Input: part model. Units: mm. Frame: model coordinates. Face numbers are marked on the shaded views. A direction names the side the tool comes from. Round coordinates to 2 decimals unless told otherwise and drop trailing zeros. Loops run counter-clockwise (first coordinate to the right, second up) from the corner with the lowest first, then second, coordinate; pieces in that order, holes last. Notation, with made-up numbers: (21.5, -36) -> (49.5, -36) arc R20 cw to (49.5, -18) -> close; hole circle Ø10 at (32, 25.5). An arc over 180 degrees is marked (long way). One line per question, with ' | ' between items. Start each with the question number.
Q1. Material intervals for L1, parallel to Z at x = 0, y = 4.05; L2, parallel to X at y = 3.25, z = -1; L3, parallel to Y at x = -2.5, z = 0.2, sorted ascending.
Q2. Cut plane C-C on z = 2.45. Return loops of the section in (x, y), and give its area (3 significant figures).
Q3. Access query for the marked faces 4 and 5. Directions: +Z, -Z, +X, -X, +Y, -Y. A direction counts if a zero-diameter tool reaches every point of the face in a straight line with its end or side. Return the directions, or none.
Q4. Contact query for a flat-ended pin moving along its axis: P1, Ø3, axis at y = 4, z = -2, coming from the -X side. Output: stop coordinate, or through.
Q5. Cut plane B-B on z = -2.15. Return loops of the section in (x, y).
Q6. Cut plane A-A on y = 4.75. Return loops of the section in (x, z).
Q7. Mould query, pull axis Z, two halves, no side actions, for the marked faces 1, 2 and 3. Classes: pulls with the +Z half, pulls with the -Z half, needs draft (parallel to the pull), parting line crosses it, or undercut.
from build123d import *

# Parameters (mm, degrees)
BOSS_EXTRUDE1_DEPTH       = 6
SKETCH2_R                 = 1.5
BOSS_EXTRUDE2_DEPTH       = 5
M3X0_5_TAPPED_HOLE1_D     = 2.5
M3X0_5_TAPPED_HOLE1_DEPTH = 5.5
M3X0_5_TAPPED_HOLE1_TIP   = 0.751075774


with BuildPart() as part:
    # Sketch1 → Boss-Extrude1 (new body)
    with BuildSketch(Plane(origin=(0, 0, 0), x_dir=(1, 0, 0), z_dir=(0, 1, 0))):
        Polygon((1.58771324, 2.75), (-1.58771324, 2.75), (-3.175426481, 0), (-1.58771324, -2.75), (1.58771324, -2.75), (3.175426481, 0), align=None)
    extrude(amount=BOSS_EXTRUDE1_DEPTH)

    # Sketch2 → Boss-Extrude2 (add)
    with BuildSketch(Plane.XZ):
        with Locations(Location((0, 0, 0), (0, 0, 90))):
            Circle(SKETCH2_R)
    extrude(amount=BOSS_EXTRUDE2_DEPTH)

    # M3x0.5 Tapped Hole1
    with Locations(Plane(origin=(0, 6, 0), x_dir=(1, 0, 0), z_dir=(0, 1, 0))):
        with Locations((0, 0)):
            Hole(M3X0_5_TAPPED_HOLE1_D / 2, depth=M3X0_5_TAPPED_HOLE1_DEPTH)
            with Locations((0, 0, -(M3X0_5_TAPPED_HOLE1_DEPTH + M3X0_5_TAPPED_HOLE1_TIP / 2))):  # 118° drill point
                Cone(0, M3X0_5_TAPPED_HOLE1_D / 2, M3X0_5_TAPPED_HOLE1_TIP, mode=Mode.SUBTRACT)


solid = part.part
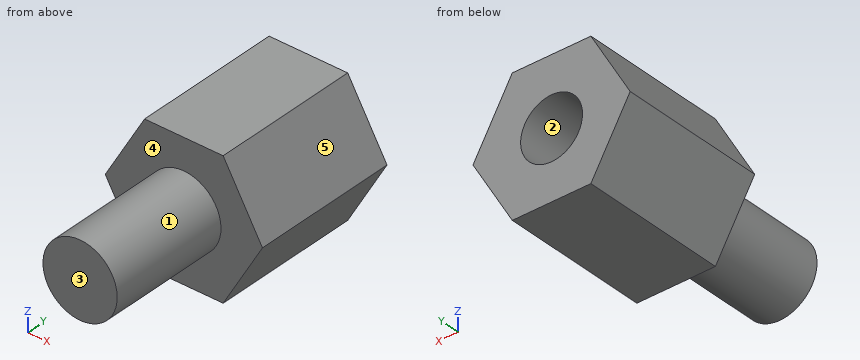
Results:
1) L1: -2.75 to -1.25, 1.25 to 2.75 | L2: -2.6 to -0.75, 0.75 to 2.6 | L3: 0 to 6
2) outline: (-1.76, 0) -> (1.76, 0) -> (1.76, 6) -> (-1.76, 6) -> close | area: 21.1 mm^2
3) face 4: -Y | face 5: +Z, +X, +Y, -Y
4) P1: x = -2.89
5) outline: (-1.93, 0) -> (1.93, 0) -> (1.93, 6) -> (-1.93, 6) -> close
6) outline: (-3.18, 0) -> (-1.59, -2.75) -> (1.59, -2.75) -> (3.18, 0) -> (1.59, 2.75) -> (-1.59, 2.75) -> close; hole circle Ø2.5 at (0, 0)
7) face 1: parting line crosses it | face 2: undercut | face 3: needs draft
